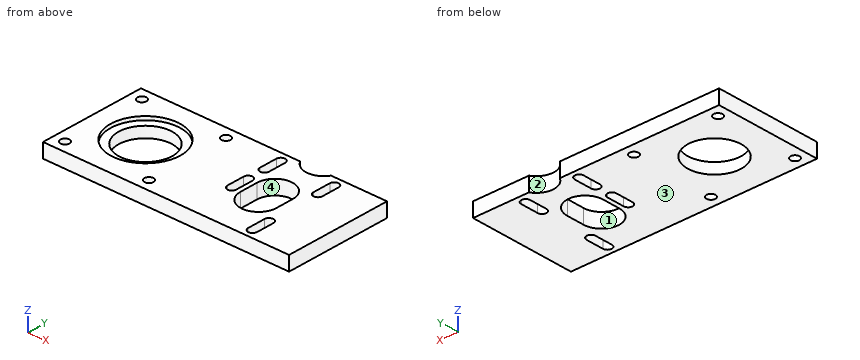
Autodesk Inventor part; units mm, degrees
ref_plane "YZ Plane" through (0, 0, 0) normal (1, 0, 0) x (0, 1, 0)
ref_plane "XZ Plane" through (0, 0, 0) normal (0, 1, 0) x (-1, 0, 0)
ref_plane "XY Plane" through (0, 0, 0) normal (0, 0, 1) x (1, 0, 0)
sketch "Szkic1" plane through (0, 0, 0) normal (0, 0, 1) x (1, 0, 0)
  arc A0 (89.3398, 60) -> (106.6602, 60) centre (98, 65.0001) ccw
  line L0 (70, 60) -> (89.3398, 60)
  line L1 (70, 0) -> (70, 60)
  line L2 (70, 0) -> (138, 0)
  line L3 (138, 60) -> (138, 0)
  line L4 (106.6602, 60) -> (138, 60)
  line L5 (80.5, 25) -> (80.5, 35)
  arc A1 (85.5, 35) -> (80.5, 35) centre (83, 35) ccw
  line L6 (85.5, 35) -> (85.5, 25)
  arc A2 (80.5, 25) -> (85.5, 25) centre (83, 25) ccw
  line L7 (115.5, 55) -> (115.5, 45)
  arc A3 (110.5, 45) -> (115.5, 45) centre (113, 45) ccw
  line L8 (110.5, 45) -> (110.5, 55)
  arc A4 (115.5, 55) -> (110.5, 55) centre (113, 55) ccw
  line L9 (80.5, 45) -> (80.5, 55)
  arc A5 (85.5, 55) -> (80.5, 55) centre (83, 55) ccw
  line L10 (85.5, 55) -> (85.5, 45)
  arc A6 (80.5, 45) -> (85.5, 45) centre (83, 45) ccw
  line L11 (115.5, 15) -> (115.5, 5)
  arc A7 (110.5, 5) -> (115.5, 5) centre (113, 5) ccw
  line L12 (110.5, 5) -> (110.5, 15)
  arc A8 (115.5, 15) -> (110.5, 15) centre (113, 15) ccw
  line L13 (88, 25) -> (88, 35)
  arc A9 (108, 35) -> (88, 35) centre (98, 35) ccw
  line L14 (108, 35) -> (108, 25)
  arc A10 (88, 25) -> (108, 25) centre (98, 25) ccw
  circle A11 centre (30, 30) radius 19.5
  circle A12 centre (53.57, 53.57) radius 2.5
  circle A13 centre (6.43, 6.43) radius 2.5
  circle A14 centre (6.43, 53.57) radius 2.5
  circle A15 centre (53.57, 6.43) radius 2.5
  line L15 (70, 60) -> (70, 0)
  line L16 (0, 60) -> (70, 60)
  line L17 (0, 0) -> (0, 60)
  line L18 (70, 0) -> (0, 0)
  circle A16 centre (30, 30) radius 15
  point P0 (35, 30)
extrude "Wyciągnięcie proste1" add sketch "Szkic1" along normal blind 8 contours A0 L4 L3 L2 L1 L0 | L1 L18 L17 L16
sketch "Szkic2" plane through (0, 0, 0) normal (0, 0, -1) x (-1, 0, 0)
  circle A0 centre (-30, 30) radius 15
  circle A1 centre (-30, 30) radius 19.5
  point P0 (0, 0)
extrude "Wyciągnięcie proste2" add sketch "Szkic2" against normal blind 6
thread "Gwint1"
thread "Gwint2"
thread "Gwint3"
thread "Gwint4"
properties part number "Uchwyt silnika krokowego osi X - płaski"
Model file for the job. Use its own axes, mm. Face numbers are marked on the shaded views. Coordinates: 2 decimals unless noted, no trailing zeros. Loops run counter-clockwise (first coordinate to the right, second up) from the corner with the lowest first, then second, coordinate; pieces in that order, holes last. Notation, with made-up numbers: (-17.75, 72) - (30.25, 72) arc R25 cw to (30.25, 97) - close; hole circle Ø1 at (20.5, 34.25). An arc over 180 degrees is marked (long way). Answer as a JSON object with one key per item and string values. Group by question number.
(1) Flat gauge pins, fed straight in: pin 1 (3 mm diameter, centred on x = 6.43, y = 6.43, fed in from -Z); pin 2 (4 mm diameter, centred on x = 20, y = 20, fed in from +Z). Where does each tip first touch, or does it go through?
(2) Two-plate mould, pull along Y, no slides. Class the marked faces 1, 2, 3 and 4: released by +Y, released by -Y, zero draft, split by the parting line, or undercut.
(3) Cut at A-A (x = 6.43). Give the cut face in (y, z).
(4) Probe line 1 along Y through (x, z) = (53.57, 5.75); line 2 along X through (y, z) = (48, 5.75); line 3 along X through (y, z) = (13, 3). List the from-to ranges inside material, lowest first.
(5) Cut at C-C (z = 3.5). State how many separate pieces and enclosed holes the cut face has, then the cut area to 3 significant figures.
(6) Cut at D-D (x = 30). Give the cut face in (y, z), then the cut area to 3 significant figures.
(7) Cut at B-B (y = 6.43). Give the cut face in (x, z).
Geometry says:
{
 "1": {"pin 1": "passes through", "pin 2": "stops at z = 6"},
 "2": {"face 1": "undercut", "face 2": "released by +Y", "face 3": "zero draft", "face 4": "undercut"},
 "3": {"outline": "(0, 0) - (3.93, 0) - (3.93, 8) - (0, 8) - close; (8.93, 0) - (51.07, 0) - (51.07, 8) - (8.93, 8) - close; (56.07, 0) - (60, 0) - (60, 8) - (56.07, 8) - close"},
 "4": {"line 1": "y = 0 to 3.93, 8.93 to 51.07, 56.07 to 60", "line 2": "x = 0 to 80.5, 85.5 to 110.5, 115.5 to 138", "line 3": "x = 0 to 110.5, 115.5 to 138"},
 "5": {"separate pieces": "1", "enclosed holes": "10", "area": "6,640 mm^2"},
 "6": {"outline": "(0, 0) - (15, 0) - (15, 6) - (10.5, 6) - (10.5, 8) - (0, 8) - close; (45, 0) - (60, 0) - (60, 8) - (49.5, 8) - (49.5, 6) - (45, 6) - close", "area": "222 mm^2"},
 "7": {"outline": "(0, 0) - (3.93, 0) - (3.93, 8) - (0, 8) - close; (8.93, 0) - (51.07, 0) - (51.07, 8) - (8.93, 8) - close; (56.07, 0) - (110.5, 0) - (110.5, 8) - (56.07, 8) - close; (115.5, 0) - (138, 0) - (138, 8) - (115.5, 8) - close"}
}
